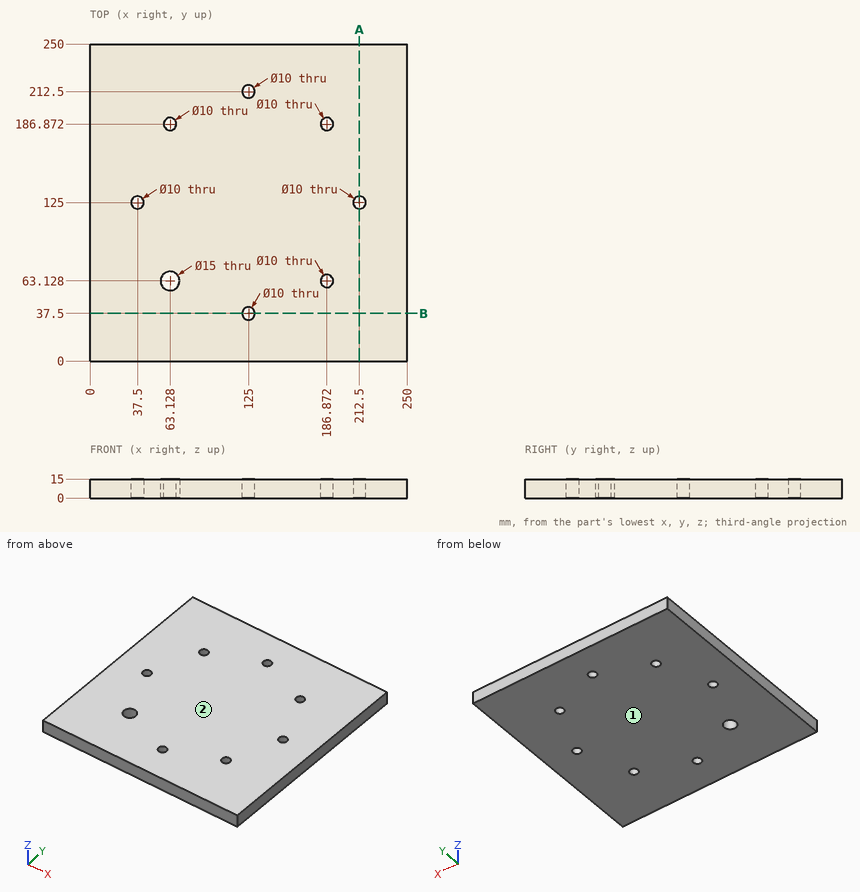
Design review of the part shown in the three views and the two pictorial views. Dimensions are in mm from the part's minimum x, y and z. Give positions to 0.01 mm unless a question says otherwise; leave off trailing zeros. Loops run counter-clockwise (first coordinate to the right, second up) from the corner with the lowest first, then second, coordinate; pieces in that order, holes last. Notation, with made-up numbers: M 49.5,66.25 L 104.5,66.25 A34 ccw 104.5,97.25 Z; hole C -20,89.5 d7. An arc over 180 degrees is marked long. Put each result on its own line as item: value. Start each with the question number.
(1) Wall thickness on L1, parallel to Y at x = 212.5, z = 4.5; L2, parallel to Y at x = 65, z = 13.75 (1 decimal): over which ranges is each line inside the solid? List them lowest first.
(2) Add section A-A, the plane x = 212.5. Write out the cut boundary in (y, z).
(3) The part is to be moulded in two halves that separate along Z. For the marked faces 1 and 2, say which applies: +Z half, -Z half, draft (parallel to the pull), parting line (faces both ways), or undercut.
Result:
1. L1: y = 0 to 120, 130 to 250
1. L2: y = 0 to 55.9, 70.4 to 182.2, 191.5 to 250
2. outline: M 0,0 L 120,0 L 120,15 L 0,15 Z; M 130,0 L 250,0 L 250,15 L 130,15 Z
3. face 1: -Z half
3. face 2: +Z half
